The model under review builds one solid part; all positions refer to its coordinate system, in mm. A direction names the side the tool comes from. Round coordinates to 2 decimals unless told otherwise and drop trailing zeros. Order: outer loops, then holes, each group sorted by start corner. A loop starts at its lowest first (then second) coordinate and runs counter-clockwise, first axis right, second up.
```python
from build123d import *

# Parameters (mm, degrees)
F0_W     = 17
F0_H     = 17
F1_DEPTH = 5
F3_DEPTH = 3
F4_R     = 5.25
F5_DEPTH = 25
F7_DEPTH = 8.5


with BuildPart() as f1:
    # F0 (on Top) → F1 (new body)
    with BuildSketch(Plane.XY):
        Rectangle(F0_W, F0_H)
    extrude(amount=F1_DEPTH)

    # F2 (on face) → F3 (cut)
    with BuildSketch(Plane.XY.offset(5)):
        Polygon((6.5, 6.5), (-6.5, 6.5), (-6.5, -6.5), (-5, -6.5), (-5, -8.5), (5, -8.5), (5, -6.5), (6.5, -6.5), align=None)
    extrude(amount=-F3_DEPTH, mode=Mode.SUBTRACT)

    # F4 (on face) → F5 (cut)
    with BuildSketch(Plane(origin=(0, 0, 0), x_dir=(1, 0, 0), z_dir=(0, 0, -1))):
        Circle(F4_R)
    extrude(amount=-F5_DEPTH, mode=Mode.SUBTRACT)

    # F6 (on Right) → F7 (join, symmetric)
    with BuildSketch(Plane.YZ):
        Polygon((8.5, 5), (8.5, 0), (17.480478, 0), (13.139273, 24.620194), (8.46825, 23.796566), (11.782592, 5), align=None)
    extrude(amount=F7_DEPTH, both=True)


solid = f1.part
```
(1) To check wall thickness, follow probe 1 along X at (y, z) = (0, 1.35); probe 2 along Z at (x, y) = (7.5, -7); probe 3 along Z at (x, y) = (4, 5.5). State the ranges of each line that lie inside material, in increasing order.
Data:
probe 1: x = -8.5 to -5.25, 5.25 to 8.5
probe 2: z = 0 to 5
probe 3: z = 0 to 2
(2) For faces 1 (the flat face through (5, -8, 4)), 2 (the cylindrical face through (5, -1.6, 1)), 3 (the flat face through (-6.5, 0, 4)), list the 3-axis set-ups (+Z, -Z, +X, -X, +Y, -Y) from which the entire face can be reached by the end or side of a thin tool; tool diameter is ignored.
Data:
face 1: +Z, -Y
face 2: +Z, -Z
face 3: +Z
(3) Consider section A-A (y = 0). Write out the cut boundary in (x, z).
Data:
outline: (-8.5, 0) - (-5.25, 0) - (-5.25, 2) - (-6.5, 2) - (-6.5, 5) - (-8.5, 5) - close; (5.25, 0) - (8.5, 0) - (8.5, 5) - (6.5, 5) - (6.5, 2) - (5.25, 2) - close
(4) Consider section B-B (x = 0). Write out the cut boundary in (y, z), and give its area (3 significant figures).
Data:
outline: (-8.5, 0) - (-5.25, 0) - (-5.25, 2) - (-8.5, 2) - close; (5.25, 0) - (17.48, 0) - (13.14, 24.62) - (8.47, 23.8) - (11.78, 5) - (6.5, 5) - (6.5, 2) - (5.25, 2) - close
area: 154 mm2
(5) Consider section D-D (z = 18.75). Write out the cut boundary in (x, y), and give its area (3 significant figures).
Data:
outline: (-8.5, 9.36) - (8.5, 9.36) - (8.5, 14.17) - (-8.5, 14.17) - close
area: 81.9 mm2
(6) Insertion check: pin 1 (3 mm diameter, centred on x = 4, z = 8.5, fed in from -Y); pin 2 (6 mm diameter, centred on x = -1.5, z = 10, fed in from -Y); pin 3 (1.2 mm diameter, centred on x = 6, z = 3.5, fed in from +Y); pin 4 (4 mm diameter, centred on x = -2.5, y = -0.5, fed in from +Z). Each pin has a flat end and moves straight along its axis. Give the tip position at first contact, or say it passes through.
Data:
pin 1: stops at y = 10.9
pin 2: stops at y = 10.37
pin 3: stops at y = 16.97
pin 4: passes through
(7) Draft analysis for pull direction Z (two halves, no side actions). For faces 4 (the flat face through (0.119, 10.102, 14.53)), 5 (the flat face through (0, 9, 5)), 6 (the flat face through (0, 7, 0)), 7 (the flat face through (0, -8.5, 1)), state which applies: pulls with the +Z half, pulls with the -Z half, needs draft (parallel to the pull), parting line crosses it, or undercut.
Data:
face 4: undercut
face 5: undercut
face 6: pulls with the -Z half
face 7: needs draft
(8) Consider section C-C (x = 5.75). Write out the cut boundary in (y, z), and give its area (3 significant figures).
Data:
outline: (-8.5, 0) - (17.48, 0) - (13.14, 24.62) - (8.47, 23.8) - (11.78, 5) - (6.5, 5) - (6.5, 2) - (-6.5, 2) - (-6.5, 5) - (-8.5, 5) - close
area: 181 mm2
